```python
from build123d import *

# Parameters (mm, degrees)
CROQUIS1_W                  = 180
CROQUIS1_H                  = 129.33
SALIENTE_EXTRUIR1_DEPTH     = 50
CORTAR_EXTRUIR1_REACH       = 167.307
CORTAR_EXTRUIR2_REACH       = 199.691
VACIADO1_T                  = -4
SALIENTE_EXTRUIR4_DEPTH     = 102.58126129
CORTAR_EXTRUIR10_DEPTH      = 92.58126129
CROQUIS15_W                 = 55.421449745
CROQUIS15_H                 = 50
CORTAR_EXTRUIR11_DEPTH      = 146.33724632
CORTAR_EXTRUIR11_DEPTH_BACK = 146.33724632
SALIENTE_EXTRUIR6_REACH     = 181.671
CROQUIS19_W                 = 20
CROQUIS19_H                 = 20
CROQUIS20_W                 = 20
CROQUIS20_H                 = 5
CORTAR_EXTRUIR14_DEPTH      = 8
CORTAR_EXTRUIR15_REACH      = 121.61
CROQUIS22_R                 = 1.585


with BuildPart() as part:
    # Croquis1 → Saliente-Extruir1 (new body)
    with BuildSketch(Plane(origin=(0, 0, 0), x_dir=(1, 0, 0), z_dir=(0, 1, 0))):
        Rectangle(CROQUIS1_W, CROQUIS1_H)
    extrude(amount=SALIENTE_EXTRUIR1_DEPTH)

    # Croquis2 → Cortar-Extruir1 (cut, up to next)
    with BuildSketch(Plane.XY.offset(64.665), mode=Mode.PRIVATE) as cortar_extruir1_sk1:
        Polygon((90, 0), (54.98962309, 50), (90, 50), align=None)
    cortar_extruir1_tool1 = extrude(cortar_extruir1_sk1.sketch, amount=-CORTAR_EXTRUIR1_REACH, mode=Mode.PRIVATE) & part.part
    cortar_extruir1 = cortar_extruir1_tool1.solids().sort_by_distance((78.329874, 33.333333, 64.665))[0]
    add(cortar_extruir1, mode=Mode.SUBTRACT)

    # Cortar-Extruir2: up to this plane
    cortar_extruir2_end = Plane(origin=(90, 0, -64.666), z_dir=(-0.819152044288995, -0.5735764363510416, 0))
    # Croquis4 → Cortar-Extruir2 (cut, up to the surface)
    with BuildSketch(Plane.ZY.offset(90), mode=Mode.PRIVATE) as cortar_extruir2_sk1:
        Polygon((-64.665, 0), (-29.65462309, 50), (-64.665, 50), align=None)
    cortar_extruir2_tool1 = split(extrude(cortar_extruir2_sk1.sketch, amount=-CORTAR_EXTRUIR2_REACH, mode=Mode.PRIVATE), bisect_by=cortar_extruir2_end, keep=Keep.BOTH, mode=Mode.PRIVATE)
    cortar_extruir2 = cortar_extruir2_tool1.solids().sort_by_distance((-90, 33.333333, -52.994874))[0]
    add(cortar_extruir2, mode=Mode.SUBTRACT)

    # Simetría2: Cortar-Extruir2 across plane
    add(cortar_extruir2.mirror(Plane.XY), mode=Mode.SUBTRACT)

    # Simetría1: Cortar-Extruir1 across plane
    add(cortar_extruir1.mirror(Plane(origin=(0, 0, 0), x_dir=(0, 0, 1), z_dir=(1, 0, 0))), mode=Mode.SUBTRACT)

    # Simetría1 at the second plane: Cortar-Extruir1 across plane
    add(cortar_extruir1.mirror(Plane.XY), mode=Mode.SUBTRACT)

    # Vaciado1
    vaciado1_openings = [part.faces().sort_by_distance(p)[0] for p in [
        (0, 0, 0),
    ]]
    offset(amount=VACIADO1_T, openings=vaciado1_openings, kind=Kind.INTERSECTION)

    # Croquis7 → Saliente-Extruir4 (add)
    with BuildSketch(Plane(origin=(0, 14.764441718, 0), x_dir=(-1, 0, 0), z_dir=(0, 0, -1))):
        Polygon((-54.98962309, 10.235558282), (-72.494811545, 10.235558282), (-54.98962309, 35.235558282), (54.98962309, 35.235558282), (72.494811545, 10.235558282), (54.98962309, 10.235558282), align=None)
    extrude(amount=SALIENTE_EXTRUIR4_DEPTH)

    # Croquis14 → Cortar-Extruir10 (cut)
    with BuildSketch(Plane.XY):
        Polygon((-85.116901645, 0), (-52.87991258, 46.039191676), (52.934417466, 46.039191676), (85.116901645, 0), align=None)
    extrude(amount=-CORTAR_EXTRUIR10_DEPTH, mode=Mode.SUBTRACT)

    # Croquis15 → Cortar-Extruir11 (cut, two sides)
    with BuildSketch(Plane(origin=(0, 0, 0), x_dir=(0, 0, -1), z_dir=(1, 0, 0))) as cortar_extruir11_sk:
        with Locations((74.870536418, 25)):
            Rectangle(CROQUIS15_W, CROQUIS15_H)
    extrude(amount=CORTAR_EXTRUIR11_DEPTH, mode=Mode.SUBTRACT)
    extrude(cortar_extruir11_sk.sketch, amount=-CORTAR_EXTRUIR11_DEPTH_BACK, mode=Mode.SUBTRACT)

    # Croquis19 → Saliente-Extruir6 (add, up to next)
    with BuildSketch(Plane(origin=(70, 0, 0), x_dir=(0, 0, -1), z_dir=(1, 0, 0)), mode=Mode.PRIVATE) as saliente_extruir6_sk1:
        with Locations((-1.703719293, 10)):
            Rectangle(CROQUIS19_W, CROQUIS19_H)
    saliente_extruir6_tool1 = extrude(saliente_extruir6_sk1.sketch, amount=SALIENTE_EXTRUIR6_REACH, mode=Mode.PRIVATE) - part.part
    saliente_extruir6 = saliente_extruir6_tool1.solids().sort_by_distance((70, 10, 1.703719))[0]
    add(saliente_extruir6)

    # Croquis20 → Cortar-Extruir14 (cut)
    with BuildSketch(Plane.ZY.offset(-70)):
        with Locations((1.703719293, 7.5)):
            Rectangle(CROQUIS20_W, CROQUIS20_H)
    cortar_extruir14 = extrude(amount=-CORTAR_EXTRUIR14_DEPTH, mode=Mode.SUBTRACT)

    # Croquis22 → Cortar-Extruir15 (cut, up to next)
    with BuildSketch(Plane(origin=(0, 5, 0), x_dir=(1, 0, 0), z_dir=(0, 1, 0)), mode=Mode.PRIVATE) as cortar_extruir15_sk1:
        with Locations(Location((74, -1.703719293, 0), (0, 0, 270))):
            Circle(CROQUIS22_R)
    cortar_extruir15_tool1 = extrude(cortar_extruir15_sk1.sketch, amount=-CORTAR_EXTRUIR15_REACH, mode=Mode.PRIVATE) & part.part
    cortar_extruir15 = cortar_extruir15_tool1.solids().sort_by_distance((74, 5, 1.703719))[0]
    add(cortar_extruir15, mode=Mode.SUBTRACT)

    # Simetría3: Saliente-Extruir6, Cortar-Extruir14, Cortar-Extruir15 across plane
    add(saliente_extruir6.mirror(Plane(origin=(0, 0, 0), x_dir=(0, 0, 1), z_dir=(1, 0, 0))))
    add(cortar_extruir14.mirror(Plane(origin=(0, 0, 0), x_dir=(0, 0, 1), z_dir=(1, 0, 0))), mode=Mode.SUBTRACT)
    add(cortar_extruir15.mirror(Plane(origin=(0, 0, 0), x_dir=(0, 0, 1), z_dir=(1, 0, 0))), mode=Mode.SUBTRACT)


solid = part.part
```
Design review of the part built by this model. Coordinates are the model's own, in mm. A direction names the side the tool comes from. Give positions to 0.01 mm unless a question says otherwise; leave off trailing zeros. Order: outer loops, then holes, each group sorted by start corner. A loop starts at its lowest first (then second) coordinate and runs counter-clockwise, first axis right, second up. Notation, with made-up numbers: (25.5, -4) -> (29.5, -4) arc R24 cw to (29.5, 13) -> close; hole circle Ø11 at (-5.75, 10.25). An arc over 180 degrees is marked (long way). Write each question's results on one line, items separated by ' | '. Start each with the question number.
Q1. Add section B-B on y = 39. Give the boundary of the cut face in (x, z).
Q2. Add section C-C on z = -16. Give the boundary of the cut face in (x, y), and give its area (3 significant figures).
Q3. Wall thickness on L1, parallel to Z at x = 74, y = 1.85; L2, parallel to Z at x = 74, y = 1.6; L3, parallel to X at y = 27, z = 29: over which ranges is each line inside the solid? List them lowest first. Write a range as from..to.
Q4. Machinability: for faces 5 (the flat face through (-70, 15, 2)), 6 (the flat face through (0, 47, -47.16)), 7 (the flat face through (-76, 5, 2)), which of the approach directions +Z, -Z, +X, -X, +Y, -Y give a long, thin tool a straight path to every point of the face, cutting with its end or side? Answer none if there is none.
Q5. For pin 1 (8 mm diameter, centred on x = 7, y = 31, fed in from -Z); pin 2 (16.5 mm diameter, centred on x = 76.5, y = 15, fed in from +Z); pin 3 (8 mm diameter, centred on x = -28, y = 30, fed in from -Z); pin 4 (3 mm diameter, centred on x = 57.5, y = 38, fed in from -Z), all flat-tipped, find the tip position at first contact; note any pin that passes through.
Q6. Mouldability with a two-part tool opening along Z and no side actions: class faces 1 (the flat face through (76, 3, -8.296)), 2 (the flat face through (76, 3, 11.704)), 3 (the flat face through (-76, 3, 11.704)), 4 (the flat face through (76, 5, 2)) as +Z half, -Z half, draft (parallel to the pull), parting line (faces both ways), or undercut.
Q7. Add section A-A on x = -19. Give the boundary of the cut face in (y, z) (3 decimals).
Found:
1) outline: (-62.69, -47.16) -> (-57.81, -47.16) -> (-57.81, 32.47) -> (57.81, 32.47) -> (57.81, 0) -> (57.85, 0) -> (57.85, -47.16) -> (62.69, -47.16) -> (62.69, 37.36) -> (-62.69, 37.36) -> close
2) outline: (-90, 0) -> (-85.12, 0) -> (-52.88, 46.04) -> (52.93, 46.04) -> (85.12, 0) -> (90, 0) -> (54.99, 50) -> (-54.99, 50) -> close | area: 895 mm2
3) L1: z = -8.3..0.12, 3.29..11.7, 58.49..63.37 | L2: z = -8.3..0.12, 3.29..11.7, 58.66..63.54 | L3: x = -71.09..-66.21, 66.21..71.09
4) face 5: -Z, -Y | face 6: -Z, +X, -X, +Y, -Y | face 7: -Z
5) pin 1: stops at z = 35.27 | pin 2: stops at z = 59.94 | pin 3: stops at z = 35.97 | pin 4: stops at z = -47.16
6) face 1: -Z half | face 2: undercut | face 3: undercut | face 4: draft
7) outline: (0, 59.782) -> (46, 27.572) -> (46, 0) -> (46.039, 0) -> (46.039, -47.16) -> (50, -47.16) -> (50, 29.655) -> (0, 64.665) -> close
